```python
from build123d import *

# Parameters (mm, degrees)
F1_DEPTH       = 8
F2_DEPTH       = 4
F4_D           = 3.3
F4_CBORE_D     = 6.5
F4_CBORE_DEPTH = 3


with BuildPart() as f1:
    # F0 (on Top) → F1 (new body)
    with BuildSketch(Plane.XY):
        with BuildLine():
            Line((0, 40), (0, 32))
            ThreePointArc((0, 32), (12.5, 32.4116301035), (25, 32))
            Line((25, 32), (25, 40))
            ThreePointArc((25, 40), (12.5, 52.5), (0, 40))
        make_face()
    extrude(amount=F1_DEPTH)

    # F0 (on Top) → F2 (join)
    with BuildSketch(Plane.XY):
        with BuildLine():
            Line((0, 32), (0, 5))
            ThreePointArc((0, 5), (1.4644660941, 1.4644660941), (5, 0))
            Line((5, 0), (20, 0))
            ThreePointArc((20, 0), (23.5355339059, 1.4644660941), (25, 5))
            Line((25, 5), (25, 32))
            ThreePointArc((25, 32), (12.5, 32.4116301035), (0, 32))
        make_face()
    extrude(amount=F2_DEPTH)

    # F4 (through all)
    with Locations(Plane.XY.offset(8)):
        with Locations((12.5, 40)):
            CounterBoreHole(F4_D / 2, F4_CBORE_D / 2, F4_CBORE_DEPTH)


solid = f1.part
```
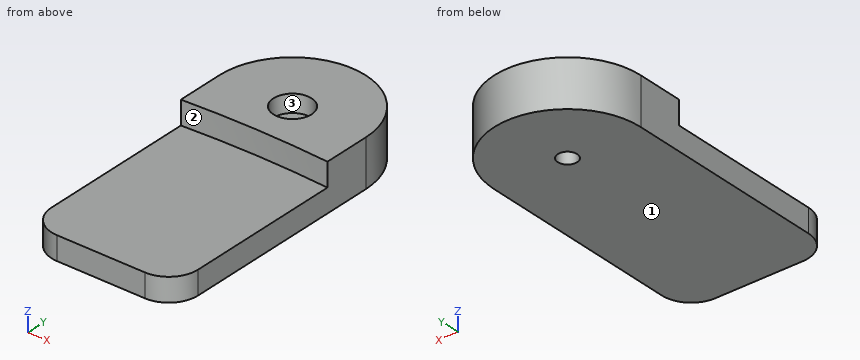
Can you work these out from the model? Positions are in its coordinate system, mm. Face numbers are marked on the shaded views. A direction names the side the tool comes from. Give positions to 0.01 mm unless a question says otherwise; leave off trailing zeros. Loops run counter-clockwise (first coordinate to the right, second up) from the corner with the lowest first, then second, coordinate; pieces in that order, holes last. Notation, with made-up numbers: M 36,55.5 L 41,55.5 A11 ccw 41,74.5 Z; hole C -16.75,67 d11. An arc over 180 degrees is marked long. One line per question, with ' | ' between items. Start each with the question number.
Q1. If we section it at C-C (y = 21.5): Please give me the cut outline in (x, z).
Q2. If I drill on line 1 (Y direction, x = 12.5, z = 7.1); line 2 (Y direction, x = 12.5, z = 2.1); line 3 (Z direction, x = 3.5, y = 12.5), over which ranges is the centre line in solid material (lowest first)? Write a range as from..to.
Q3. If we section it at D-D (z = 6.25): Please give me the cut outline in (x, y).
Q4. For the marked faces 1, 2 and 3, which set-ups out of +Z, -Z, +X, -X, +Y, -Y let a thin tool reach every point of the face, with its end or its side?
Q5. If we section it at A-A (x = 12.5): Please give me the cut outline in (y, z).
Q6. If we section it at B-B (z = 1.25): Please give me the cut outline in (x, y).
Q7. For pin 1 Ø2 at (x, y) = (13, 39.5) entering from +Z; pin 2 Ø6 at (x, y) = (15.5, 18.5) entering from +Z; pin 3 Ø3 at (x, y) = (12.5, 40) entering from -Z; pin 4 Ø1.5 at (x, z) = (3.5, 4.5) entering from -Y, each with a flat end and sliding along its axis, tell me the tip position at first contact or that it passes through.
Computed:
1) outline: M 0,0 L 25,0 L 25,4 L 0,4 Z
2) line 1: y = 32.41..36.75, 43.25..52.5 | line 2: y = 0..38.35, 41.65..52.5 | line 3: z = 0..4
3) outline: M 0,32 A190 cw 25,32 L 25,40 A12.5 ccw 0,40 Z; hole C 12.5,40 d6.5
4) face 1: -Z, +X, -X, +Y, -Y | face 2: +Z, -Y | face 3: +Z
5) outline: M 0,0 L 38.35,0 L 38.35,5 L 36.75,5 L 36.75,8 L 32.41,8 L 32.41,4 L 0,4 Z; M 41.65,0 L 52.5,0 L 52.5,8 L 43.25,8 L 43.25,5 L 41.65,5 Z
6) outline: M 0,5 A5 ccw 5,0 L 20,0 A5 ccw 25,5 L 25,40 A12.5 ccw 0,40 Z; hole C 12.5,40 d3.3
7) pin 1: stops at z = 5 | pin 2: stops at z = 4 | pin 3: passes through | pin 4: stops at y = 0.09
